Geometry check sheet. Reference: the model listing, model coordinates, mm. A direction names the side the tool comes from. Coordinates: 2 decimals unless noted, no trailing zeros. Order: outer loops, then holes, each group sorted by start corner. A loop starts at its lowest first (then second) coordinate and runs counter-clockwise, first axis right, second up. Notation, with made-up numbers: (66.25, -21.75) - (95.25, -21.75) arc R22 cw to (95.25, -11.75) - close; hole circle Ø5 at (5, 64.5). An arc over 180 degrees is marked (long way). Put each result on its own line as item: value.
Autodesk Inventor part; units mm, degrees
ref_plane "YZ Plane" through (0, 0, 0) normal (1, 0, 0) x (0, 1, 0)
ref_plane "XZ Plane" through (0, 0, 0) normal (0, 1, 0) x (-1, 0, 0)
ref_plane "XY Plane" through (0, 0, 0) normal (0, 0, 1) x (1, 0, 0)
sketch "Sketch1" plane through (0, 0, 0) normal (1, 0, 0) x (0, 1, 0)
  line L0 (0, 8) -> (-3, 8)
  line L1 (-3, 8) -> (-3, 13)
  line L2 (-3, 13) -> (0, 13)
  line L3 (0, 17) -> (0, 13)
  line L4 (0, 8) -> (0, 0)
  line L5 (148, 13) -> (151, 13)
  line L6 (151, 13) -> (151, 8)
  line L7 (151, 8) -> (148, 8)
  line L8 (148, 0) -> (148, 8)
  line L9 (148, 13) -> (148, 17)
  line L10 (30, 0) -> (30, 6)
  line L11 (30, 6) -> (40, 6)
  line L12 (40, 6) -> (40, 0)
  line L13 (108, 0) -> (108, 6)
  line L14 (108, 6) -> (118, 6)
  line L15 (118, 6) -> (118, 0)
  line L16 (40, 0) -> (108, 0)
  line L17 (148, 17) -> (0, 17)
  line L18 (30, 0) -> (0, 0)
  line L19 (118, 0) -> (148, 0)
  dimension "d1" = 148
  dimension "d2" = 5
  dimension "d3" = 3
  dimension "d7" = 10
  dimension "d9" = 30
  dimension "d31" = 6
  dimension "d38" = 17
  dimension "d39" = 8
  dimension "d40" = 2
extrude "Extrusion2" add sketch "Sketch1" along normal blind 3
properties part number "Electronics Chassis Wall"
Q1. Draft check along Y on faces 1 (the flat face through (1, -1, 8)), 2 (the flat face through (1, 0, 15)), 3 (the flat face through (1, 108, 3)). Enter one of: pulls with the +Y half, pulls with the -Y half, needs draft (parallel to the pull), parting line crosses it, or undercut.
Answer block:
face 1: needs draft
face 2: pulls with the -Y half
face 3: undercut
Q2. Access from +Z, -Z, +X, -X, +Y, -Y to the whole of each face (thin tool, end or side, straight path). Record for faces 4 (the flat face through (1, 150, 8)), 5 (the flat face through (1, 118, 3)), 6 (the flat face through (1, -2, 13)), 7 (the flat face through (1, 0, 4)), 8 (the flat face through (1, 148, 15)).
Answer block:
face 4: -Z, +X, -X, +Y
face 5: -Z, +X, -X
face 6: +Z, +X, -X, -Y
face 7: -Z, +X, -X, -Y
face 8: +Z, +X, -X, +Y
Q3. Thickness scan on L1, parallel to Y at x = 0.7, z = 5; L2, parallel to Z at x = 2, y = 109.5; L3, parallel to Y at x = 2.6, z = 16.25. Record the ranges inside material, lowest first. Write a range as [from, to].
Answer block:
L1: y = [0, 30], [40, 108], [118, 148]
L2: z = [6, 17]
L3: y = [0, 148]
Q4. Section check B-B on x = 1.8. Record the boundary of the cut face in (y, z).
Answer block:
outline: (-3, 8) - (0, 8) - (0, 0) - (30, 0) - (30, 6) - (40, 6) - (40, 0) - (108, 0) - (108, 6) - (118, 6) - (118, 0) - (148, 0) - (148, 8) - (151, 8) - (151, 13) - (148, 13) - (148, 17) - (0, 17) - (0, 13) - (-3, 13) - close
Q5. Section check C-C on z = 15. Record the boundary of the cut face in (x, y), then the cut area to 3 significant figures.
Answer block:
outline: (0, 0) - (3, 0) - (3, 148) - (0, 148) - close
area: 444 mm^2
Q6. Section check D-D on y = 38.5. Record the boundary of the cut face in (x, z), then the cut area to 3 significant figures.
Answer block:
outline: (0, 6) - (3, 6) - (3, 17) - (0, 17) - close
area: 33.0 mm^2
Q7. Section check A-A on z = 4.5. Record the boundary of the cut face in (x, y), then the cut area to 3 significant figures.
Answer block:
outline: (0, 0) - (3, 0) - (3, 30) - (0, 30) - close; (0, 40) - (3, 40) - (3, 108) - (0, 108) - close; (0, 118) - (3, 118) - (3, 148) - (0, 148) - close
area: 384 mm^2
Q8. Depth check by flat-ended pin: pin 1 Ø0.9 at (x, y) = (2, 113.5) entering from -Z; pin 2 Ø8 at (y, z) = (21, 14) entering from -X; pin 3 Ø1.5 at (x, z) = (1.5, 15.5) entering from +Y; pin 4 Ø0.9 at (x, z) = (1.5, 4) entering from -Y. Enter the tip coordinate at first touch or a pass-through.
Answer block:
pin 1: stops at z = 6
pin 2: stops at x = 0
pin 3: stops at y = 148
pin 4: stops at y = 0
